Geometry: final body of the model. Coordinates: model frame, mm. A direction names the side the tool comes from. Give positions to 0.01 mm unless a question says otherwise; leave off trailing zeros. Order: outer loops, then holes, each group sorted by start corner. A loop starts at its lowest first (then second) coordinate and runs counter-clockwise, first axis right, second up. Notation, with made-up numbers: (39.25, -24) -> (63.25, -24) arc R38 ccw to (63.25, 14) -> close; hole circle Ø11 at (47, 89). An arc over 180 degrees is marked (long way). Write item = value, one per line.
```python
from build123d import *

# Parameters (mm, degrees)
F0_W     = 15.75
F0_H     = 7.76
F1_DEPTH = 3.16
F2_R     = 2.45
F3_DEPTH = 1.75
F4_T     = -1.55
F5_R     = 1.55
F5_R_2   = 0.695
F6_DEPTH = 1.6


with BuildPart() as f1:
    # F0 (on Front) → F1 (new body)
    with BuildSketch(Plane.XZ):
        with Locations((8.467483707, 3.5795439035)):
            Rectangle(F0_W, F0_H)
    extrude(amount=-F1_DEPTH)

    # F2 (on face) → F3 (join)
    with BuildSketch(Plane.XZ):
        with Locations((4.497483707, 3.6045439035)):
            Circle(F2_R)
        with Locations((12.437483707, 3.6045439035)):
            Circle(F2_R)
    extrude(amount=F3_DEPTH)

    # F4
    f4_openings = [f1.faces().sort_by_distance(p)[0] for p in [
        (8.467484, 3.16, 3.579544),
    ]]
    offset(amount=F4_T, openings=f4_openings, kind=Kind.INTERSECTION)

    # F5 (on face) → F6 (join)
    with BuildSketch(Plane(origin=(0, 1.55, 0), x_dir=(-1, 0, 0), z_dir=(0, 1, 0))):
        with Locations((-8.467483707, 3.5795439035)):
            Circle(F5_R)
        with Locations((-8.467483707, 3.5795439035)):
            Circle(F5_R_2, mode=Mode.SUBTRACT)
    extrude(amount=F6_DEPTH)


solid = f1.part
```
1) Reachability of faces 5 (the face through (12, -1.75, 4)), 6 (the face through (8, 0, 4)), 7 (the face through (14.792, 2, 4)) from +Z, -Z, +X, -X, +Y, -Y: full face, straight path, thin tool, end or side. Return the list, or none.
Check sheet entries:
face_5 = +Z, -Z, +X, -X, -Y
face_6 = -Y
face_7 = +Y
2) Line query: line 1 (Z direction, x = 11.25, y = 1.9); line 2 (Z direction, x = 4.5, y = 0.5); line 3 (X direction, y = 2, z = 4.5). Output: solid intervals per line, ascending. Write a range as from..to.
Check sheet entries:
line_1 = -0.3..1.25, 5.91..7.46
line_2 = -0.3..2.7, 4.5..7.46
line_3 = 0.59..2.14, 7.22..9.71, 14.79..16.34
3) Mould query, pull axis X, two halves, no side actions, for faces 1 (the face through (7, 1.55, 5)), 2 (the face through (14.774, -0.863, 4.34)), 3 (the face through (4, -1.75, 4)), 4 (the face through (0.592, 2, 4)). Classes: +X half, -X half, draft (parallel to the pull), parting line (faces both ways), or undercut.
Check sheet entries:
face_1 = undercut
face_2 = undercut
face_3 = draft
face_4 = -X half
4) Section query D-D (y = 0.5). Output: boundary loops of the cut face in (x, z).
Check sheet entries:
outline = (0.59, -0.3) -> (16.34, -0.3) -> (16.34, 7.46) -> (0.59, 7.46) -> close; hole circle Ø1.8 at (4.5, 3.6); hole circle Ø1.8 at (12.44, 3.6)
5) Section query B-B (x = 4.5). Output: boundary loops of the cut face in (y, z), plus the area to 3 significant figures.
Check sheet entries:
outline = (-1.75, 1.15) -> (0, 1.15) -> (0, -0.3) -> (3.16, -0.3) -> (3.16, 1.25) -> (1.55, 1.25) -> (1.55, 2.7) -> (-0.2, 2.7) -> (-0.2, 4.5) -> (1.55, 4.5) -> (1.55, 5.91) -> (3.16, 5.91) -> (3.16, 7.46) -> (0, 7.46) -> (0, 6.05) -> (-1.75, 6.05) -> close
area = 22.4 mm²
6) First-contact query: P1, Ø1.1, axis at x = 8.47, z = 3.58, coming from the -Y side; P2, Ø1.5, axis at x = 4.5, z = 5, coming from the +Y side; P3, Ø1.5, axis at y = -1, z = 5, coming from the +X side. Flat tips, straight axial feed; report the tip coordinate or a pass-through.
Check sheet entries:
P1 = 0
P2 = 1.55
P3 = 14.8
7) Section query A-A (y = 2.2). Output: boundary loops of the cut face in (x, z) (3 decimals).
Check sheet entries:
outline = (0.592, -0.3) -> (16.342, -0.3) -> (16.342, 7.46) -> (0.592, 7.46) -> close; circle Ø3.1 at (8.467, 3.58); hole (2.142, 1.25) -> (14.792, 1.25) -> (14.792, 5.91) -> (2.142, 5.91) -> close; hole circle Ø1.39 at (8.467, 3.58)
8) Section query C-C (z = 4.75). Output: boundary loops of the cut face in (x, y), plus the area to 3 significant figures.
Check sheet entries:
outline = (0.59, 0) -> (2.33, 0) -> (2.33, -1.75) -> (6.66, -1.75) -> (6.66, 0) -> (10.27, 0) -> (10.27, -1.75) -> (14.6, -1.75) -> (14.6, 0) -> (16.34, 0) -> (16.34, 3.16) -> (14.79, 3.16) -> (14.79, 1.55) -> (9.48, 1.55) -> (9.48, 3.15) -> (7.45, 3.15) -> (7.45, 1.55) -> (2.14, 1.55) -> (2.14, 3.16) -> (0.59, 3.16) -> close
area = 47.8 mm²
